Input: part model. Units: mm. Frame: model coordinates. A direction names the side the tool comes from. Coordinates: 2 decimals unless noted, no trailing zeros. Loops run counter-clockwise (first coordinate to the right, second up) from the corner with the lowest first, then second, coordinate; pieces in that order, holes last.
(1) Set-up query: faces 1 (the face through (17.5, 0, 2)), 2 (the face through (-17.5, 0, 2)), 3 (the face through (1, -15, 5)). Return all of +Z, -Z, +X, -X, +Y, -Y with unobstructed straight access to the full face (end or side cutting, diameter ignored); none if empty.
(2) Section A-A, the plane y = -19. Return loops of the section in (x, z) (3 decimals), then the cut area to 3 significant figures.
(3) Section B-B, the plane x = -40.5. Return loops of the section in (y, z).
(4) Section C-C, the plane z = 1.5. Return loops of the section in (x, y), then the cut area to 3 significant figures.
(5) Section D-D, the plane x = -7. Return loops of the section in (y, z), then the cut area to 3 significant figures.
(6) Mould query, pull axis Y, two halves, no side actions, for faces 4 (the face through (-1, 26, 8)), 5 (the face through (1, 37, 4)), 6 (the face through (0, 0, 4)). Classes: released by +Y, released by -Y, zero draft, split by the parting line, or undercut.
(7) Contact query for flat-ended pins moving along their axis: P1, Ø5.5, axis at x = -17, y = 19, coming from the +Z side; P2, Ø2, axis at y = -7, z = 1.5, coming from the -X side; P3, Ø4, axis at x = 17, y = -19, coming from the -Z side (3 decimals); P4, Ø2, axis at y = 0, z = 2, coming from the +X side. Output: stop coordinate, or through.
(8) Line query: L1, parallel to Y at x = 17, z = 5.75; L2, parallel to Y at x = 17, z = 3.75; L3, parallel to X at y = 19, z = 5.75. Output: solid intervals per line, ascending.
```python
from build123d import *

# Parameters (mm, degrees)
EXTRUDE_1_DEPTH              = 8
SKETCH_2_W                   = 35
SKETCH_2_H                   = 30
CUT_EXTRUDE_1_DEPTH          = 4
HOLE_WIZARD_M4_1_D           = 3.3
HOLE_WIZARD_M4_1_CSINK_D     = 4.05
HOLE_WIZARD_M4_1_CSINK_ANGLE = 90
MIRROR_2_COPY_1_D            = 3.3
MIRROR_2_COPY_1_CSINK_D      = 4.05
MIRROR_2_COPY_1_CSINK_ANGLE  = 90


with BuildPart() as part:
    # 草图1 → 凸台-拉伸1 (new body)
    with BuildSketch(Plane.XY):
        Polygon((47.5, 37), (-47.5, 37), (-47.5, 15), (-17.5, 15), (-17.5, -15), (-47.5, -15), (-47.5, -37), (47.5, -37), (47.5, -15), (17.5, -15), (17.5, 15), (47.5, 15), align=None)
    extrude(amount=EXTRUDE_1_DEPTH)

    # 草图2 → 切除-拉伸1 (cut)
    with BuildSketch(Plane.XY.offset(8)):
        Rectangle(SKETCH_2_W, SKETCH_2_H)
    extrude(amount=-CUT_EXTRUDE_1_DEPTH, mode=Mode.SUBTRACT)

    # M4 螺纹孔1 (through all)
    with Locations(Plane(origin=(17, 19, 0), x_dir=(-1, 0, 0), z_dir=(0, 0, -1))):
        with Locations((0, 0)):
            hole_wizard_m4_1 = CounterSinkHole(HOLE_WIZARD_M4_1_D / 2, HOLE_WIZARD_M4_1_CSINK_D / 2, counter_sink_angle=HOLE_WIZARD_M4_1_CSINK_ANGLE)

    # 镜向1: M4 螺纹孔1 across plane
    add(hole_wizard_m4_1.mirror(Plane.ZX), mode=Mode.SUBTRACT)

    # 镜向2: M4 螺纹孔1 across plane
    add(hole_wizard_m4_1.mirror(Plane(origin=(0, 0, 0), x_dir=(0, 0, 1), z_dir=(1, 0, 0))), mode=Mode.SUBTRACT)

    # 镜向2 copy 1 (through all)
    with Locations(Plane(origin=(-17, -19, 0), x_dir=(1, 0, 0), z_dir=(0, 0, -1))):
        with Locations((0, 0)):
            CounterSinkHole(MIRROR_2_COPY_1_D / 2, MIRROR_2_COPY_1_CSINK_D / 2, counter_sink_angle=MIRROR_2_COPY_1_CSINK_ANGLE)


solid = part.part
```
Report:
1. face 1: +Z, -Z, +X
1. face 2: +Z, -Z, -X
1. face 3: +Z
2. outline: (-47.5, 0) - (-19.025, 0) - (-18.65, 0.375) - (-18.65, 8) - (-47.5, 8) - close; (-15.35, 0.375) - (-14.975, 0) - (14.975, 0) - (15.35, 0.375) - (15.35, 8) - (-15.35, 8) - close; (18.65, 0.375) - (19.025, 0) - (47.5, 0) - (47.5, 8) - (18.65, 8) - close
2. area: 707 mm2
3. outline: (-37, 0) - (-15, 0) - (-15, 8) - (-37, 8) - close; (15, 0) - (37, 0) - (37, 8) - (15, 8) - close
4. outline: (-47.5, -37) - (47.5, -37) - (47.5, -15) - (17.5, -15) - (17.5, 15) - (47.5, 15) - (47.5, 37) - (-47.5, 37) - (-47.5, 15) - (-17.5, 15) - (-17.5, -15) - (-47.5, -15) - close; hole circle Ø3.3 at (-17, -19); hole circle Ø3.3 at (-17, 19); hole circle Ø3.3 at (17, -19); hole circle Ø3.3 at (17, 19)
4. area: 5,200 mm2
5. outline: (-37, 0) - (37, 0) - (37, 8) - (15, 8) - (15, 4) - (-15, 4) - (-15, 8) - (-37, 8) - close
5. area: 472 mm2
6. face 4: zero draft
6. face 5: released by +Y
6. face 6: undercut
7. P1: stops at z = 8
7. P2: stops at x = -17.5
7. P3: stops at z = 0.025
7. P4: stops at x = 17.5
8. L1: y = -37 to -20.65, -17.35 to -15, 15 to 17.35, 20.65 to 37
8. L2: y = -37 to -20.65, -17.35 to 17.35, 20.65 to 37
8. L3: x = -47.5 to -18.65, -15.35 to 15.35, 18.65 to 47.5
